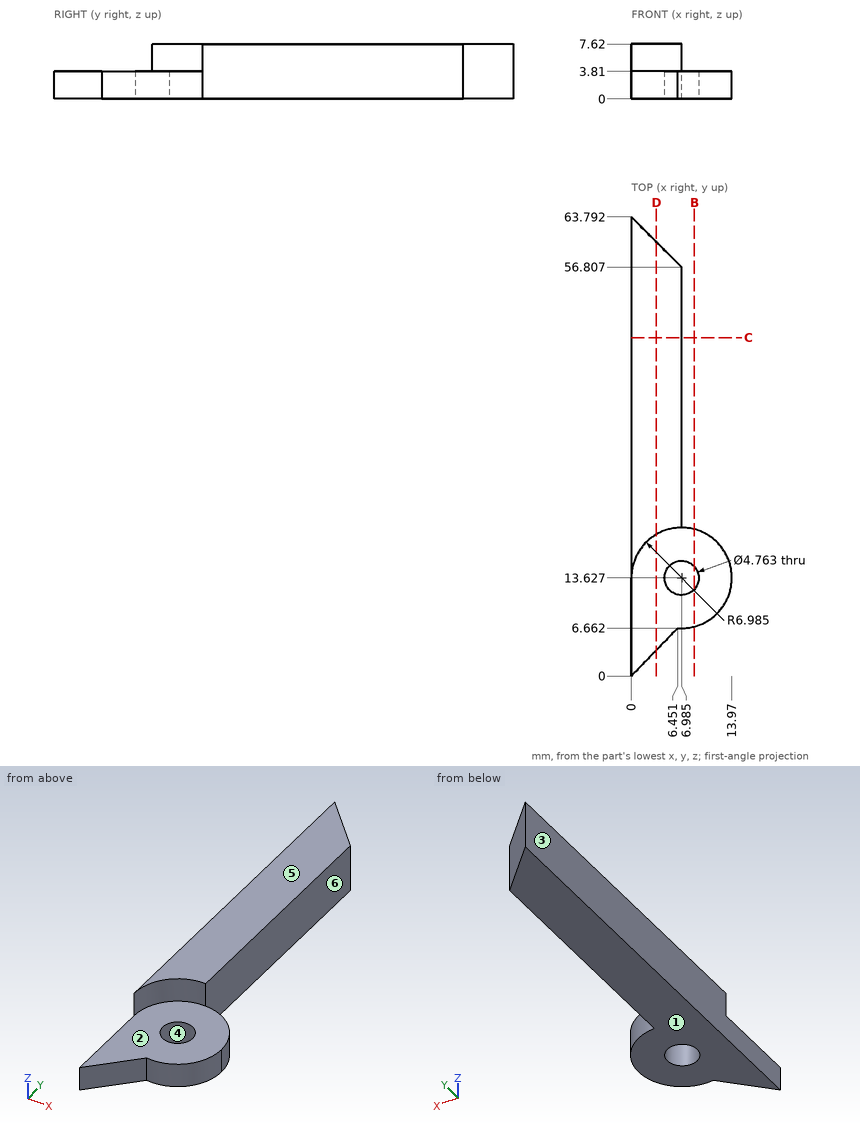
Verification items for this drawing (mm, ordinates from the low corner). A direction names the side the tool comes from. Give positions to 0.01 mm unless a question says otherwise; leave off trailing zeros. Write each loop counter-clockwise with the first axis right and the second up, starting at its lowest first coordinate (ties: lowest second). Pieces come first, ordered by that corner, then holes.
1) Thickness scan on line 1 (Z direction, x = 6.75, y = 7); line 2 (X direction, y = 32, z = 2) (1 decimal); line 3 (Y direction, x = 7.75, z = 3.75) (1 decimal). Record the ranges inside material, lowest first.
Values follow:
line 1: z = 0 to 3.81
line 2: x = 0 to 7
line 3: y = 6.7 to 11.4, 15.9 to 20.6
2) Release check for a two-part mould opening along X. For the marked faces 3, 4, 5 and 6 record: released by +X, released by -X, zero draft, split by the parting line, or undercut.
Values follow:
face 3: released by -X
face 4: undercut
face 5: zero draft
face 6: released by +X
3) Set-up check for the marked faces 1 and 2: record each of +Z, -Z, +X, -X, +Y, -Y from which the full face is reachable in a straight line by a thin tool's end or side.
Values follow:
face 1: -Z, +X, -X, +Y, -Y
face 2: +Z, +X, -Y
4) Cross-section at C-C (y = 47). Record the boundary of the cut face in (x, z) (1 decimal).
Values follow:
outline: (0, 0) - (7, 0) - (7, 7.6) - (0, 7.6) - close
5) Cross-section at D-D (x = 3.5). Record the boundary of the cut face in (y, z) (1 decimal).
Values follow:
outline: (3.6, 0) - (60.3, 0) - (60.3, 7.6) - (19.7, 7.6) - (19.7, 3.8) - (3.6, 3.8) - close
6) Go/stop test with a flat-tipped pin: pin 1 Ø3 at (x, z) = (10, 2.5) entering from -Y. Record where the tip stops, or that it passes through.
Values follow:
pin 1: stops at y = 6.81
7) Cross-section at B-B (x = 8.75). Record the boundary of the cut face in (y, z) (1 decimal).
Values follow:
outline: (6.9, 0) - (12, 0) - (12, 3.8) - (6.9, 3.8) - close; (15.2, 0) - (20.4, 0) - (20.4, 3.8) - (15.2, 3.8) - close
